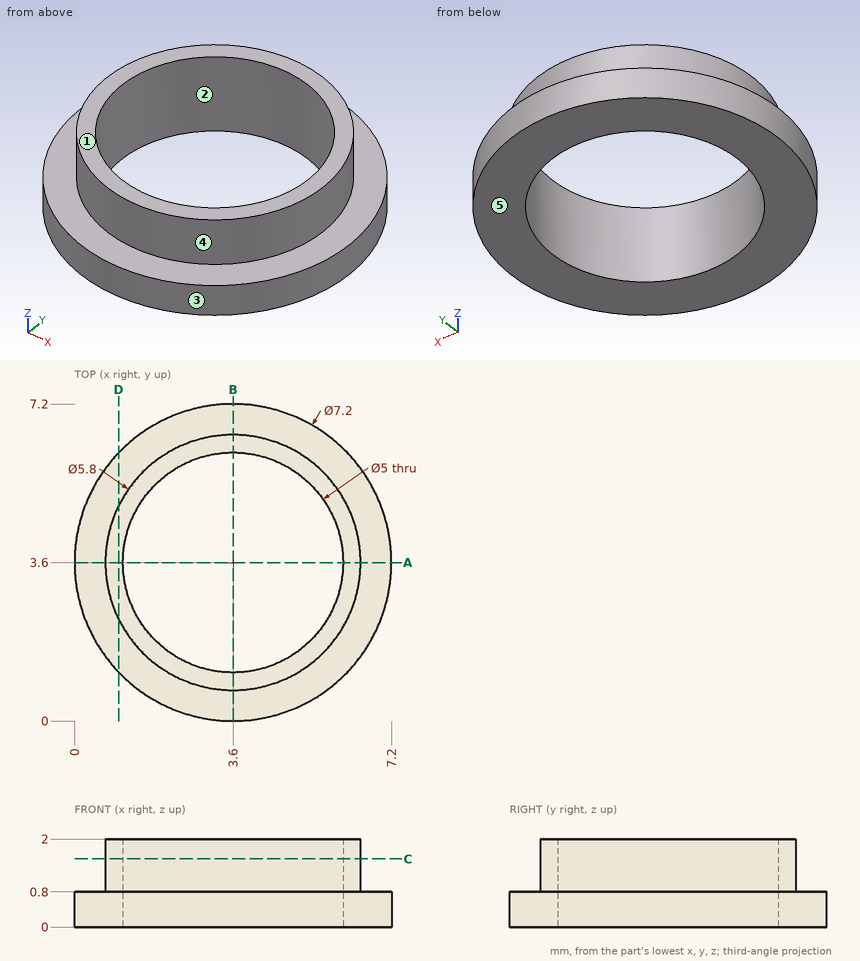
For this review, use the dimensioned drawing (mm, ordinates from the lowest corner) and the shaded views. A direction names the side the tool comes from. Round coordinates to 2 decimals unless told otherwise and drop trailing zeros. Write each loop counter-clockwise with the first axis right and the second up, starting at its lowest first coordinate (ties: lowest second). Pieces come first, ordered by that corner, then holes. Notation, with made-up numbers: (46.25, 73.25) -> (65.25, 73.25) arc R16 ccw to (65.25, 77.25) -> close; hole circle Ø4 at (33.25, 75.5). An arc over 180 degrees is marked (long way). One line per item, written item: value. Start each with the question number.
Q1. Add section C-C (z = 1.55). Give the boundary of the cut face in (x, y), then the cut area to 3 significant figures.
Q2. The part is to be moulded in two halves that separate along X. For the marked faces 1, 2 and 3, say which applies: pulls with the +X half, pulls with the -X half, needs draft (parallel to the pull), parting line crosses it, or undercut.
Q3. To check wall thickness, follow probe 1 along Y at (x, z) = (3.6, 1.65); probe 2 along Y at (x, z) = (3.5, 0.75); probe 3 along X at (y, z) = (4.25, 0.25). State the ranges of each line that lie inside material, in increasing order.
Q4. Add section A-A (y = 3.6). Give the boundary of the cut face in (x, z).
Q5. Add section D-D (x = 1). Give the boundary of the cut face in (y, z), then the cut area to 3 significant figures.
Q6. Tool access review of the marked faces 4 and 5: name each direction out of +Z, -Z, +X, -X, +Y, -Y from which nothing blocks a thin tool from reaching the whole face with its end or side.
Response:
1. outline: circle Ø5.8 at (3.6, 3.6); hole circle Ø5 at (3.6, 3.6)
1. area: 6.79 mm^2
2. face 1: needs draft
2. face 2: undercut
2. face 3: parting line crosses it
3. probe 1: y = 0.7 to 1.1, 6.1 to 6.5
3. probe 2: y = 0 to 1.1, 6.1 to 7.2
3. probe 3: x = 0.06 to 1.19, 6.01 to 7.14
4. outline: (0, 0) -> (1.1, 0) -> (1.1, 2) -> (0.7, 2) -> (0.7, 0.8) -> (0, 0.8) -> close; (6.1, 0) -> (7.2, 0) -> (7.2, 0.8) -> (6.5, 0.8) -> (6.5, 2) -> (6.1, 2) -> close
5. outline: (1.11, 0) -> (6.09, 0) -> (6.09, 0.8) -> (4.88, 0.8) -> (4.88, 2) -> (2.32, 2) -> (2.32, 0.8) -> (1.11, 0.8) -> close
5. area: 7.07 mm^2
6. face 4: +Z
6. face 5: -Z, +X, -X, +Y, -Y
